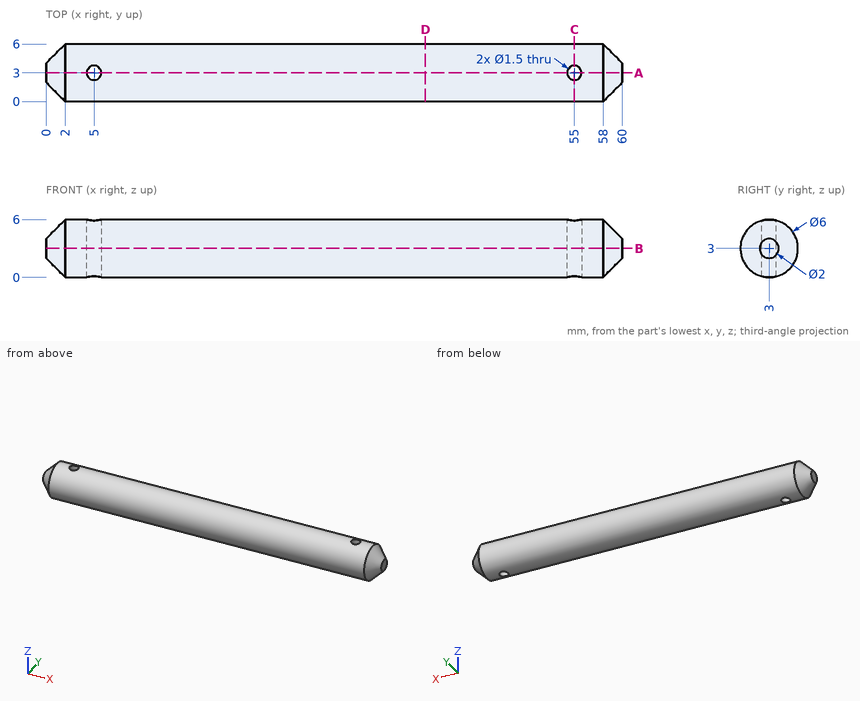
Verification items for this drawing (mm, ordinates from the low corner). Coordinates: 2 decimals unless noted, no trailing zeros. Write each loop counter-clockwise with the first axis right and the second up, starting at its lowest first coordinate (ties: lowest second). Pieces come first, ordered by that corner, then holes. Notation, with made-up numbers: M -13.5,7.25 L 13.5,7.25 A17 ccw 13.5,38.25 Z; hole C 4.5,-10.75 d10. An arc over 180 degrees is marked long. Use CSV: the item, a comma, the result in double quotes.
Q1. Section check C-C, the plane x = 55. Enter the section's corners in (y, z).
Computed values:
outline,"M 2.25,0.1 L 2.25,5.9 A3 ccw Z; M 3.75,0.1 A3 ccw 3.75,5.9 Z"
Q2. Go/stop test with flat-tipped pins: P1, Ø3, axis at x = 8.5, y = 2, coming from the -Z side; P2, Ø0.9, axis at x = 55, y = 3, coming from the +Z side; P3, Ø3, axis at x = 36, y = 5, coming from the +Z side. Record where each tip stops, or that it passes through.
Computed values:
P1,"z = 0"
P2,"through"
P3,"z = 5.96"
Q3. Section check D-D, the plane x = 39.5. Enter the section's corners in (y, z), and give its area (3 significant figures).
Computed values:
outline,"C 3,3 d6"
area,"28.3 mm²"
Q4. Section check B-B, the plane z = 3. Enter the section's corners in (x, y), and give its area (3 significant figures).
Computed values:
outline,"M 0,2 L 2,0 L 58,0 L 60,2 L 60,4 L 58,6 L 2,6 L 0,4 Z; hole C 5,3 d1.5; hole C 55,3 d1.5"
area,"348 mm²"
Q5. Thickness scan on line 1 along Y through (x, z) = (5, 3); line 2 along X through (y, z) = (3.25, 3.5); line 3 along Y through (x, z) = (55, 4). Record the ranges inside material, lowest first. Write a range as [from, to].
Computed values:
line 1,"[0, 2.25], [3.75, 6]"
line 2,"[0, 4.29], [5.71, 54.29], [55.71, 60]"
line 3,"[0.17, 2.25], [3.75, 5.83]"
Q6. Section check A-A, the plane y = 3. Enter the section's corners in (x, z).
Computed values:
outline,"M 0,2 L 2,0 L 4.25,0 L 4.25,6 L 2,6 L 0,4 Z; M 5.75,0 L 54.25,0 L 54.25,6 L 5.75,6 Z; M 55.75,0 L 58,0 L 60,2 L 60,4 L 58,6 L 55.75,6 Z"
